For this review, take the finished solid that the model builds, in its own axes (mm). A direction names the side the tool comes from. Round coordinates to 2 decimals unless told otherwise and drop trailing zeros. Write each loop counter-clockwise with the first axis right and the second up, starting at its lowest first coordinate (ties: lowest second). Pieces come first, ordered by that corner, then holes.
Autodesk Fusion 360 part; units mm, degrees
sketch "Sketch1" plane through (0, 0, 0) normal (0, 0, 1) x (1, 0, 0)
  line L0 (0, 0) -> (-130, 0)
  line L1 (-130, 0) -> (-130, 60)
  line L2 (-130, 60) -> (0, 60)
  line L3 (0, 60) -> (0, 0)
  dimension "d1" = 130
  dimension "d2" = 60
extrude "Extrude1" add sketch "Sketch1" along normal blind 38
sketch "Sketch2" plane through (0, 0, 0) normal (1, 0, 0) x (0, 1, 0)
  line L0 (0, 0) -> (60, 0)
  line L1 (60, 0) -> (60, 38)
  line L2 (60, 38) -> (0, 38)
  line L3 (0, 38) -> (0, 0)
  line L4 (30, 38) -> (13, 38)
  line L5 (30, 38) -> (47, 38)
  line L6 (13, 38) -> (13, 0)
  line L7 (13, 0) -> (45, 0)
  line L8 (45, 0) -> (47, 0)
  line L9 (47, 38) -> (47, 0)
  dimension "d5" = 17
  dimension "d6" = 17
  dimension "d7" = 2
extrude "Extrude2" cut sketch "Sketch2" against normal blind 20 contours L0 L2 L4 L5 L6 L7 L8 L9
sketch "Sketch3" plane through (0, 0, 38) normal (0, 0, 1) x (-1, 0, 0)
  line L0 (20, -47) -> (0, -47)
  line L1 (0, -47) -> (0, -60)
  line L2 (0, -60) -> (130, -60)
  line L3 (130, -60) -> (130, 0)
  line L4 (130, 0) -> (0, 0)
  line L5 (0, 0) -> (0, -13)
  line L6 (0, -13) -> (20, -13)
  line L7 (20, -13) -> (20, -47)
  line L8 (130, -30) -> (0, -30)
  line L9 (65, -60) -> (65, 0)
  circle A0 centre (65, -30) radius 40
  dimension "d10" = 80
extrude "Extrude3" add sketch "Sketch3" along normal blind 15 contours L4 L8 L9 A0 | L2 L8 L9 A0 | L2 A0 | L4 L8 L9 A0 | L2 L8 L9 A0 | L4 A0
sketch "Sketch4" plane through (0, 0, 0) normal (0, -1, 0) x (1, 0, 0)
  line L0 (-130, 0) -> (0, 0)
  line L1 (0, 0) -> (0, 38)
  line L2 (0, 38) -> (-38.5425, 38)
  line L3 (-38.5425, 38) -> (-91.4575, 38)
  line L4 (-91.4575, 38) -> (-130, 38)
  line L5 (-130, 38) -> (-130, 0)
  circle A0 centre (-15.0389, 22.7916) radius 7.5
  circle A1 centre (-15.0389, 22.7916) radius 15
  line L6 (-14.5606, 7.7992) -> (-51.278, 7.7992)
  line L7 (-51.278, 7.7992) -> (-130, 7.7992)
  line L8 (-130, 7.7992) -> (-130, 0)
  line L9 (-130, 0) -> (0, 0)
  line L10 (0, 0) -> (-0.0389, 22.8172)
  dimension "d13" = 15
  dimension "d14" = 30
extrude "Extrude4" cut sketch "Sketch4" against normal blind 85 contours L0 L5 A1 L6 L7 L8 L9 L10 | A0
sketch "Sketch5" plane through (0, 0, 0) normal (1, 0, 0) x (0, 1, 0)
  line L0 (13, 0) -> (13, 38)
  line L1 (13, 38) -> (0, 38)
  line L2 (0, 38) -> (0, 0)
  line L3 (0, 0) -> (13, 0)
  line L4 (0, 0) -> (62.2368, 0)
  line L5 (62.2368, 0) -> (62.2368, 22.3752)
  line L6 (62.2368, 22.3752) -> (0, 22.3752)
  line L7 (0, 22.3752) -> (0, 0)
extrude "Extrude5" cut sketch "Sketch5" against normal blind 0.04 contours L0 L2 L3 L4 L6 L7 | L0 L4 L5 L6
sketch "Sketch6" plane through (-20, 0, 0) normal (1, 0, 0) x (0, 1, 0)
  line L0 (13, 28.4163) -> (47, 28.4163)
  line L1 (47, 28.4163) -> (47, 38)
  line L2 (47, 38) -> (13, 38)
  line L3 (13, 38) -> (13, 28.4163)
  line L4 (13, 38) -> (47, 38)
  line L5 (47, 38) -> (47, 8)
  line L6 (47, 8) -> (13, 8)
  line L7 (13, 8) -> (13, 38)
extrude "Extrude6" cut sketch "Sketch6" against normal blind 15
sketch "Sketch7" plane through (0, 0, 8) normal (0, 0, 1) x (-1, 0, 0)
  line L0 (20, -13) -> (20, -47)
  line L1 (20, -47) -> (35, -47)
  line L2 (35, -47) -> (35, -13)
  line L3 (35, -13) -> (20, -13)
extrude "Extrude7" cut sketch "Sketch7" against normal blind 20
extrude "Extrude8" add 1 faces at (-35, 24.3333, 24.7385) along direction (1, 0, 0) blind 10
sketch "Sketch8" plane through (0, 0, 38) normal (0, 0, 1) x (-1, 0, 0)
  arc A0 (91.4575, -60) -> (91.4575, 0) centre (65, -30) ccw
  line L0 (91.4575, -60) -> (130, -60)
  line L1 (130, -60) -> (130, 0)
  line L2 (130, 0) -> (91.4575, 0)
  line L3 (130, -30) -> (113, -30)
  line L4 (113, -30) -> (105, -30)
  line L5 (115.0261, -30) -> (115.0261, -55)
  line L6 (115.0261, -30) -> (115.0261, -5)
  circle A1 centre (115.0261, -5) radius 3.5
  circle A2 centre (115.0261, -55) radius 3.5
  dimension "d25" = 25
  dimension "d26" = 25
  dimension "d27" = 7
  dimension "d28" = 7
extrude "Extrude9" cut sketch "Sketch8" against normal blind 80 contours A2 | A1
sketch "Sketch9" plane through (0, 0, 0) normal (0, -1, 0) x (1, 0, 0)
  line L0 (-0.0382, 22.3752) -> (0, 22.3752)
  line L1 (0, 22.3752) -> (0, 38)
  line L2 (0, 38) -> (-38.5425, 38)
  line L3 (-38.5425, 38) -> (-91.4575, 38)
  line L4 (-91.4575, 38) -> (-130, 38)
  line L5 (-130, 38) -> (-130, 7.7992)
  line L6 (-130, 7.7992) -> (-15.5172, 7.7992)
  arc A0 (-15.5172, 7.7992) -> (-0.0389, 22.8172) centre (-15.0389, 22.7916) ccw
  line L7 (-0.0389, 22.8172) -> (-0.0382, 22.3752)
  circle A1 centre (-15.0389, 22.7916) radius 7.5
  circle A2 centre (-15.0389, 22.7916) radius 15
  line L8 (-15.1827, 38) -> (0, 40)
  line L9 (0, 40) -> (2, 37)
  line L10 (2, 37) -> (2, 23.4709)
  line L11 (2, 23.4709) -> (-0.0543, 23.4709)
  line L12 (-15.1827, 38) -> (-15.1827, 37.7909)
  dimension "d31" = 30
extrude "Extrude10" cut sketch "Sketch9" against normal blind 75 contours L1 L2 A2 L11 L12 | L1 L2 L8 L9 L10 L11
sketch "Sketch10" plane through (0, 0, 53) normal (0, 0, 1) x (-1, 0, 0)
  circle A0 centre (65, -30) radius 40
  circle A1 centre (65, -30) radius 18
  line L0 (65, -30) -> (65, -48)
  line L1 (65, -30) -> (65, -12)
  line L2 (65, -12) -> (65, -21)
  line L3 (65, -12) -> (65, -21)
  line L4 (65, -12) -> (26.0256, -21)
  line L5 (65, -48) -> (65, -39)
  line L6 (65, -48) -> (26.0256, -39)
  line L7 (26.0256, -39) -> (25.172, -33.7058)
  line L8 (25.172, -33.7058) -> (25.0231, -28.6402)
  line L9 (25.0231, -28.6402) -> (25.3066, -25.057)
  line L10 (25.3066, -25.057) -> (26.0256, -21)
  dimension "d34" = 36
extrude "Extrude11" add sketch "Sketch10" along normal blind 10 contours A1 L4 L6 L7 L8 L9 L10 | A1 L0 L1 L2 L3 L4 L5 L6 | A1 L0 L1 L2 L3 L5
sketch "Sketch11" plane through (0, 0, 63) normal (0, 0, 1) x (-1, 0, 0)
  arc A0 (65, -48) -> (65, -12) centre (65, -30) ccw
  line L0 (65, -12) -> (26.0256, -21)
  line L1 (26.0256, -21) -> (25.3066, -25.057)
  line L2 (25.3066, -25.057) -> (25.0231, -28.6402)
  line L3 (25.0231, -28.6402) -> (25.172, -33.7058)
  line L4 (25.172, -33.7058) -> (26.0256, -39)
  line L5 (26.0256, -39) -> (65, -48)
  circle A1 centre (70, -25) radius 2
  circle A2 centre (70, -35) radius 2
  line L6 (68, -25) -> (72, -25)
  line L7 (72, -25) -> (72, -34.9977)
  line L8 (72, -34.9977) -> (68, -34.9977)
  line L9 (68, -34.9977) -> (68, -25)
  dimension "d37" = 4
extrude "Extrude12" cut sketch "Sketch11" against normal blind 10 contours A1 L6 | A1 A2 L7 L9 | A1 L6 | A2 L8 | A2 L8
(1) We need section A-A, the plane y = 5. State how many separate pieces and enclosed holes the cut face has, and give its area (3 significant figures).
Geometry check:
separate pieces: 2
enclosed holes: 1
area: 4,370 mm2
(2) For pin 1 Ø4 at (x, z) = (-15, 15.5) entering from -Y; pin 2 Ø20 at (x, z) = (-12.5, 24) entering from +Y; pin 3 Ø1.5 at (y, z) = (22, 38) entering from +X, all flat-tipped, find the tip position at first contact; note any pin that passes through.
Geometry check:
pin 1: stops at y = 0
pin 2: stops at y = 60
pin 3: stops at x = -25
(3) For faces 5 (the face through (-25.605, 36.39, 57.93)), 6 (the face through (-64, 0, 23)), 7 (the face through (-83, 30, 58)), 8 (the face through (-25.163, 26.874, 57.93)), list the 3-axis set-ups (+Z, -Z, +X, -X, +Y, -Y) from which the entire face can be reached by the end or side of a thin tool; tool diameter is ignored.
Geometry check:
face 5: +Z, +X, +Y
face 6: -Z, +X, -X, -Y
face 7: +Z, -X
face 8: +Z, +X, -Y
(4) We need section D-D, the plane x = -70. Give the boundary of the cut face in (y, z).
Geometry check:
outline: (-9.69, 38) - (0, 38) - (0, 7.8) - (60, 7.8) - (60, 38) - (69.69, 38) - (69.69, 53) - (47.29, 53) - (47.29, 63) - (37, 63) - (37, 53) - (23, 53) - (23, 63) - (12.71, 63) - (12.71, 53) - (-9.69, 53) - close
(5) Mouldability with a two-part tool opening along Y and no side actions: class faces 1 (the face through (-45.786, 43.563, 57.93)), 2 (the face through (-25, 30, 23)), 3 (the face through (-118.364, 53.949, 23.111)), 4 (the face through (-23, 53, 38)) as pulls with the +Y half, pulls with the -Y half, needs draft (parallel to the pull), parting line crosses it, or undercut.
Geometry check:
face 1: pulls with the +Y half
face 2: undercut
face 3: undercut
face 4: needs draft
(6) For line 1 along X through (y, z) = (56, 26.5); line 2 along Z through (x, y) = (-35, 58); line 3 along Z through (x, y) = (-46, 29.5), list the stretches that pass through material, from the lowest coordinate up.
Geometry check:
line 1: x = -130 to -118.38, -111.67 to -21.56, -8.52 to -0.5
line 2: z = 7.8 to 38
line 3: z = 7.8 to 63
(7) We need section B-B, the plane z = 18. Give the boundary of the cut face in (x, y), and give its area (3 significant figures).
Geometry check:
outline: (-130, 0) - (-20.81, 0) - (-20.81, 13) - (-25, 13) - (-25, 47) - (-20.81, 47) - (-20.81, 60) - (-130, 60) - close; (-9.27, 0) - (-0.82, 0) - (-0.82, 13) - (-9.27, 13) - close; (-9.27, 47) - (-0.82, 47) - (-0.82, 60) - (-9.27, 60) - close; hole circle Ø7 at (-115.03, 5); hole circle Ø7 at (-115.03, 55)
area: 6,550 mm2
